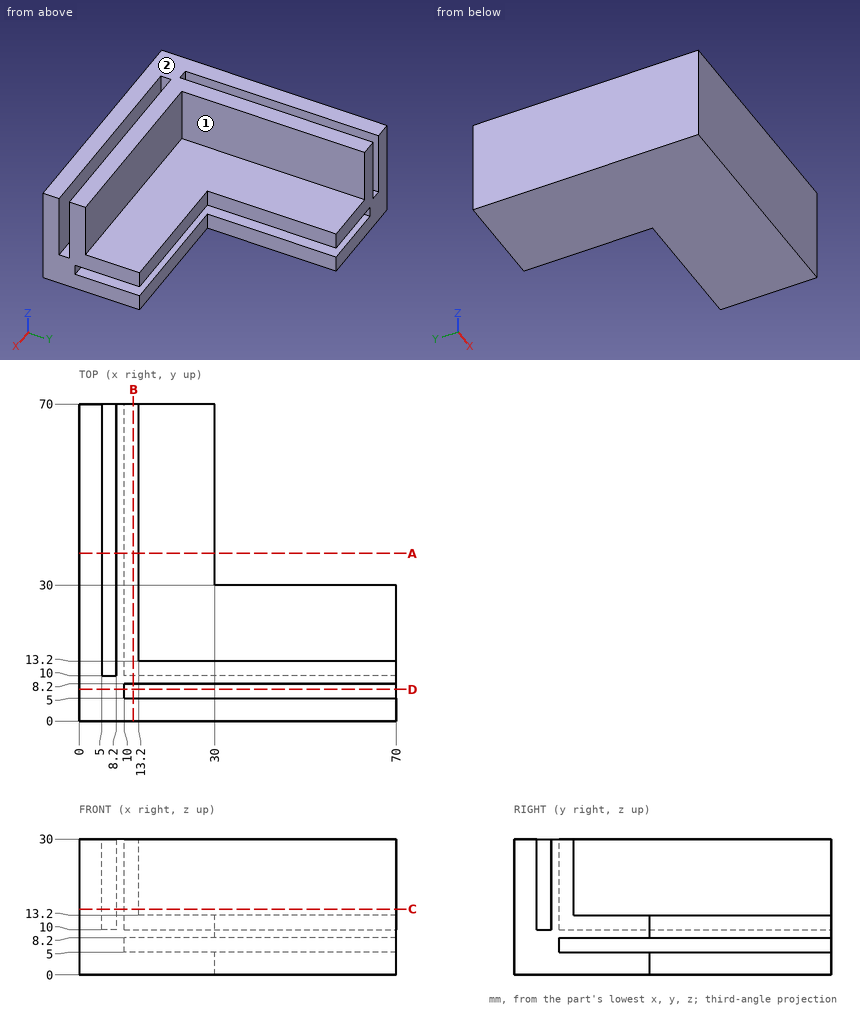
Print and shaded views of the part. All mm, measured from the part's lowest x, y and z. A direction names the side the tool comes from. Round coordinates to 2 decimals unless told otherwise and drop trailing zeros. Order: outer loops, then holes, each group sorted by start corner. A loop starts at its lowest first (then second) coordinate and runs counter-clockwise, first axis right, second up.
Q1. Drop flat-ended pins along their axis: pin 1 (2 mm diameter, centred on y = 40, z = 9, fed in from +X); pin 2 (10 mm diameter, centred on x = 35, z = 16, fed in from +Y); pin 3 (1.6 mm diameter, centred on x = 47, y = 6, fed in from +Z). Give the stop position or say it passes through.
Q2. Wall check: L1, parallel to Z at x = 12, y = 19.5; L2, parallel to X at y = 20.5, z = 25. Give the ranges that are in metal, low to high.
Q3. Slice it at A-A (y = 37). Write the cut outline in (x, z), and give its area (3 significant figures).
Q4. Slice it at B-B (x = 12). Write the cut outline in (y, z).
Q5. Slice it at C-C (z = 14.5). Write the cut outline in (x, y), and give its area (3 significant figures).
Q6. Slice it at D-D (y = 7). Write the cut outline in (x, z).
Q7. Which spindle directions (+Z, -Z, +X, -X, +Y, -Y) get a long thin tool onto all of the face, cutting with end or side? Do the marked faces 1 and 2. Say none if no direction does.
Results below:
1. pin 1: stops at x = 30
1. pin 2: stops at y = 30
1. pin 3: stops at z = 10
2. L1: z = 0 to 5, 8.2 to 30
2. L2: x = 0 to 5, 8.2 to 13.2
3. outline: (0, 0) - (30, 0) - (30, 5) - (10, 5) - (10, 8.2) - (30, 8.2) - (30, 13.2) - (13.2, 13.2) - (13.2, 30) - (8.2, 30) - (8.2, 10) - (5, 10) - (5, 30) - (0, 30) - close
3. area: 490 mm2
4. outline: (0, 0) - (70, 0) - (70, 5) - (10, 5) - (10, 8.2) - (70, 8.2) - (70, 30) - (8.2, 30) - (8.2, 10) - (5, 10) - (5, 30) - (0, 30) - close
5. outline: (0, 0) - (70, 0) - (70, 5) - (10, 5) - (10, 8.2) - (70, 8.2) - (70, 13.2) - (13.2, 13.2) - (13.2, 70) - (8.2, 70) - (8.2, 10) - (5, 10) - (5, 70) - (0, 70) - close
5. area: 1,290 mm2
6. outline: (0, 0) - (70, 0) - (70, 10) - (10, 10) - (10, 30) - (0, 30) - close
7. face 1: +Z, +X, +Y
7. face 2: +Z, +X, -X, +Y, -Y
